Autodesk Inventor part; units mm, degrees
ref_plane "MSC_PF1" through (0, 0, 0) normal (1, 0, 0) x (0, 1, 0)
ref_plane "MSC_PT1" through (0, 0, 0) normal (1, 0, 0) x (0, 1, 0)
ref_plane "YZ Plane" through (0, 0, 0) normal (1, 0, 0) x (0, 1, 0)
sketch "Skizze1" plane through (0, 0, 0) normal (0, 1, 0) x (-1, 0, 0)
  point P0 (0, 0)
sketch "Skizze2" plane through (0, 0, 0) normal (0, 0, 1) x (-1, 0, 0)
  line L0 (-8, 2.5) -> (-8, 0)
  line L1 (-2.8, 2.5) -> (-8, 2.5)
  line L2 (-0.3, 5) -> (-2.8, 2.5)
  line L3 (0, 5) -> (-0.3, 5)
  line L4 (0, 0) -> (0, 5)
  line L5 (-8, 0) -> (0, 0)
  line L6 (-8, 0) -> (0, 0)
  line L7 (0, -9.6) -> (0, 1.6)
  line L8 (1.6, 0) -> (-9.6, 0)
  dimension "ParC" = 0.3
  dimension "d43" = 45
  dimension "d44" = 5
  dimension "d45" = 2.5
  dimension "d46" = 8
  dimension "d47" = 0
  dimension "d48" = 0
revolve "Drehung1" add sketch "Skizze2" angle 360 about axis through (8, 0, 0) along (1, 0, 0)
sketch "Skizze3" plane through (0, 0, 0) normal (-1, 0, 0) x (0, 0, 1)
  line L0 (-1.5, 0.866) -> (-1.5, -0.866)
  line L1 (0, 1.7321) -> (-1.5, 0.866)
  line L2 (1.5, 0.866) -> (0, 1.7321)
  line L3 (1.5, -0.866) -> (1.5, 0.866)
  line L4 (0, -1.7321) -> (1.5, -0.866)
  line L5 (-1.5, -0.866) -> (0, -1.7321)
  circle A0 centre (0, 0) radius 1.5 construction
  circle A1 centre (0, 0) radius 2.5 construction
  dimension "d11" = 3
  dimension "d13" = 120
  dimension "d15" = 120
extrude "Extrusion1" cut sketch "Skizze3" against normal blind 2.3
fillet "Rundung1" radius 0.2 1 edges at (2.8, 2.5, 0)
chamfer "Fase1" distance 0.4 angle 45 1 edges at (8, 2.5, 0) measured on face at (6.2943, 0.599, -2.4272)
thread "Gewinde1"
ref_plane "MSC_PF1" through (0, 0, 0) normal (1, 0, 0) x (0, 1, 0)
ref_plane "MSC_PT1" through (0, 0, 0) normal (1, 0, 0) x (0, 1, 0)
equation "\"d43\" = 0.5 * ang"
equation "\"d44\" = 0.5 * dk"
equation "\"d45\" = 0.5 * NND"
equation "\"d46\" = NLG"
equation "\"d11\" = ParS"
equation "\"d16\" = ParT"
equation "\"d18\" = r"
equation "\"d19\" = 0.5 * PTC"
equation "\"d39\" = 0.5 * PTC"
equation "\"NND\" = 5"
equation "\"PTC\" = 0.8"
equation "\"ParK\" = 2.8"
equation "\"ParS\" = 3"
equation "\"ParT\" = 2.3"
equation "\"r\" = 0.2"
equation "\"NLG\" = 8"
equation "\"ang\" = 90deg"
equation "\"THREADDIA\" = NND"
properties part number "ISO 10642 - M5 x  8" material "Stahl"
Model file for the job. Use its own axes, mm. A direction names the side the tool comes from. Coordinates: 2 decimals unless noted, no trailing zeros. Order: outer loops, then holes, each group sorted by start corner. A loop starts at its lowest first (then second) coordinate and runs counter-clockwise, first axis right, second up. Notation, with made-up numbers: M 16.5,-11.5 L 37.5,-11.5 A18 cw 37.5,9.5 Z; hole C 41,-25 d8. An arc over 180 degrees is marked long. Return JSON: item names as keys, results as strings.
1. Saw through at A-A (x = 0.75). Give the cut face in (y, z).
Ans:
{"outline": "C 0,0 d9.1; hole M -1.73,0 L -0.87,-1.5 L 0.87,-1.5 L 1.73,0 L 0.87,1.5 L -0.87,1.5 Z"}
2. Flat gauge pins, fed straight in: pin 1 (1.5 mm diameter, centred on x = 2.5, y = -0.5, fed in from -Z); pin 2 (4 mm diameter, centred on x = 2.5, z = -3, fed in from -Y); pin 3 (2 mm diameter, centred on x = 4, y = 2.5, fed in from +Z). Where does each tip first touch, or does it go through?
Ans:
{"pin 1": "z = -3.52", "pin 2": "y = -4.08", "pin 3": "z = 2"}
3. Drill centre lines: probe 1 along Z at (x, y) = (0.5, -0.5); probe 2 along X at (y, z) = (-1, 0.5); probe 3 along Y at (x, z) = (3, 2). Where is each one in solid material? Low to high.
Ans:
{"probe 1": "-4.77 to -1.5, 1.5 to 4.77", "probe 2": "2.3 to 8", "probe 3": "-1.5 to 1.5"}
4. Tool access for faces 1 (the face through (2.3, 0, 0)), 2 (the face through (0, 0, 2)), 3 (the face through (5.27, 0.54, 2.44)): list every direction of +Z, -Z, +X, -X, +Y, -Y with a clear straight run to the whole face (end or side of a thin tool).
Ans:
{"face 1": "-X", "face 2": "+Z, -Z, -X, +Y, -Y", "face 3": "+X"}
5. Pull direction Y, two halves, no side cores. Call faces 4 (the face through (8, 0, 0)), 5 (the face through (2.589, -1.251, -2.405)), 6 (the face through (1.134, -1.293, -0.76)): +Y half, -Y half, draft (parallel to the pull), parting line (faces both ways), or undercut.
Ans:
{"face 4": "draft", "face 5": "parting line", "face 6": "undercut"}
6. Saw through at C-C (x = 6.25). Give the cut face in (y, z), and give its area (3 significant figures).
Ans:
{"outline": "C 0,0 d5", "area": "19.6 mm^2"}
7. Saw through at B-B (x = 1.75). Give the cut face in (y, z), and give its area (3 significant figures).
Ans:
{"outline": "C 0,0 d7.1; hole M -1.73,0 L -0.87,-1.5 L 0.87,-1.5 L 1.73,0 L 0.87,1.5 L -0.87,1.5 Z", "area": "31.8 mm^2"}
